Check sheet for the modelled part. Datum: model origin and axes. Units: mm. Face numbers are marked on the shaded views. A direction names the side the tool comes from. Round coordinates to 2 decimals unless told otherwise and drop trailing zeros. Write each loop counter-clockwise with the first axis right and the second up, starting at its lowest first coordinate (ties: lowest second). Pieces come first, ordered by that corner, then holes. Notation, with made-up numbers: M -29.75,44.5 L -4.75,44.5 A13 cw -4.75,62.5 Z; hole C 85,52.25 d9. An arc over 180 degrees is marked long. Answer in a Markdown table with one row per item.
```python
from build123d import *

# Parameters (mm, degrees)
SKETCH_W        = 50
SKETCH_H        = 50
PAD_DEPTH       = 20
POCKET_DEPTH    = 20.001
POCKET001_DEPTH = 50.001
POCKET002_DEPTH = 50.001
SKETCH009_R     = 1.55
POCKET008_DEPTH = 5


with BuildPart() as part:
    # Sketch → Pad (new body)
    with BuildSketch(Plane.XY):
        Rectangle(SKETCH_W, SKETCH_H)
    extrude(amount=PAD_DEPTH)

    # Sketch001 (on Face6 of Pad) → Pocket (cut, through all)
    with BuildSketch(Plane.XY.offset(20)):
        with BuildLine():
            Line((-18, 15), (-17, 15))
            ThreePointArc((-17, 15), (-15.585786, 15.585786), (-15, 17))
            Line((-15, 17), (-15, 18))
            ThreePointArc((-13, 20), (-14.414214, 19.414214), (-15, 18))
            Line((-13, 20), (13, 20))
            ThreePointArc((15, 18), (14.414214, 19.414214), (13, 20))
            Line((15, 18), (15, 17))
            ThreePointArc((15, 17), (15.585786, 15.585786), (17, 15))
            Line((17, 15), (18, 15))
            ThreePointArc((20, 13), (19.414214, 14.414214), (18, 15))
            Line((20, 13), (20, -13))
            ThreePointArc((18, -15), (19.414214, -14.414214), (20, -13))
            Line((18, -15), (17, -15))
            ThreePointArc((17, -15), (15.585786, -15.585786), (15, -17))
            Line((15, -17), (15, -18))
            ThreePointArc((13, -20), (14.414214, -19.414214), (15, -18))
            Line((13, -20), (-13, -20))
            ThreePointArc((-15, -18), (-14.414214, -19.414214), (-13, -20))
            Line((-15, -18), (-15, -17))
            ThreePointArc((-15, -17), (-15.585786, -15.585786), (-17, -15))
            Line((-17, -15), (-18, -15))
            ThreePointArc((-20, -13), (-19.414214, -14.414214), (-18, -15))
            Line((-20, -13), (-20, 13))
            ThreePointArc((-18, 15), (-19.414214, 14.414214), (-20, 13))
        make_face()
    extrude(amount=-POCKET_DEPTH, mode=Mode.SUBTRACT)

    # Sketch002 (on Face3 of Pocket) → Pocket001 (cut, through all)
    with BuildSketch(Plane.YZ.offset(25)):
        with BuildLine():
            Line((-15, 13), (15, 13))
            ThreePointArc((20, 8), (18.535534, 11.535534), (15, 13))
            Line((20, 8), (20, 0))
            Line((20, 0), (-20, 0))
            Line((-20, 0), (-20, 8))
            ThreePointArc((-15, 13), (-18.535534, 11.535534), (-20, 8))
        make_face()
    extrude(amount=-POCKET001_DEPTH, mode=Mode.SUBTRACT)

    # Sketch003 (on Face6 of Pocket) → Pocket002 (cut, through all)
    with BuildSketch(Plane.XZ.offset(25)):
        with BuildLine():
            Line((-15, 13), (15, 13))
            ThreePointArc((20, 8), (18.535534, 11.535534), (15, 13))
            Line((20, 8), (20, 0))
            Line((20, 0), (-20, 0))
            Line((-20, 0), (-20, 8))
            ThreePointArc((-15, 13), (-18.535534, 11.535534), (-20, 8))
        make_face()
    extrude(amount=-POCKET002_DEPTH, mode=Mode.SUBTRACT)

    # Sketch009 → Pocket008 (cut)
    with BuildSketch(Plane.XY.offset(20)):
        with Locations((-20, 20)):
            Circle(SKETCH009_R)
        with Locations((20, 20)):
            Circle(SKETCH009_R)
        with Locations((20, -20)):
            Circle(SKETCH009_R)
        with Locations((-20, -20)):
            Circle(SKETCH009_R)
    extrude(amount=-POCKET008_DEPTH, mode=Mode.SUBTRACT)


solid = part.part
```
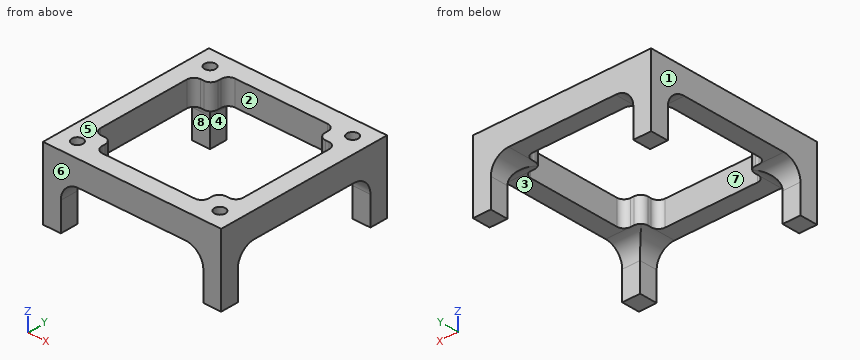
1. Draft check along X on the marked faces 1, 2 and 3. Enter one of: +X half, -X half, draft (parallel to the pull), parting line (faces both ways), or undercut.
Found:
| item | result |
|---|---|
| face 1 | -X half |
| face 2 | undercut |
| face 3 | draft |
2. Go/stop test with flat-tipped pins: pin 1 (1.6 mm diameter, centred on x = 20.5, y = -19.5, fed in from +Z); pin 2 (5 mm diameter, centred on x = -12, y = 15.5, fed in from -Z); pin 3 (5.5 mm diameter, centred on x = 3.5, y = -21.5, fed in from -Z). Record where each tip stops, or that it passes through.
Found:
| item | result |
|---|---|
| pin 1 | stops at z = 15 |
| pin 2 | passes through |
| pin 3 | stops at z = 13 |
3. Scan lines: L1, parallel to X at y = 21.5, z = 1.25; L2, parallel to X at y = -19.5, z = 17.5. Record each from-to range of solid material in increasing order.
Found:
| item | result |
|---|---|
| L1 | x = -25 to -20, 20 to 25 |
| L2 | x = -25 to -21.47, -18.53 to -14.32, 14.32 to 18.53, 21.47 to 25 |
4. Section check A-A, the plane x = 9. Record the cut outline in (y, z), and give its area (3 significant figures).
Found:
| item | result |
|---|---|
| outline | M -25,13 L -20,13 L -20,20 L -25,20 Z; M 20,13 L 25,13 L 25,20 L 20,20 Z |
| area | 70.0 mm2 |
5. Access from +Z, -Z, +X, -X, +Y, -Y to the whole of each face (thin tool, end or side, straight path). Record for the marked faces 4, 5, 6, 7 and 8.
Found:
| item | result |
|---|---|
| face 4 | -Z, +Y, -Y |
| face 5 | +Z, +X, -X, +Y, -Y |
| face 6 | +Z, -Z, +X, -X, -Y |
| face 7 | +Z, -Z |
| face 8 | -Z, +X, -X |
6. Section check D-D, the plane z = 16.5. Count the separate pieces of the cut face and the enclosed holes in it, and give its area (3 significant figures).
Found:
| item | result |
|---|---|
| separate pieces | 1 |
| enclosed holes | 5 |
| area | 973 mm2 |
7. Section check C-C, the plane z = 11. Record the cut outline in (x, y), and give its area (3 significant figures).
Found:
| item | result |
|---|---|
| outline | M -25,-25 L -19,-25 L -19,-19 L -25,-19 Z; M -25,19 L -19,19 L -19,25 L -25,25 Z; M 19,-25 L 25,-25 L 25,-19 L 19,-19 Z; M 19,19 L 25,19 L 25,25 L 19,25 Z |
| area | 144 mm2 |
